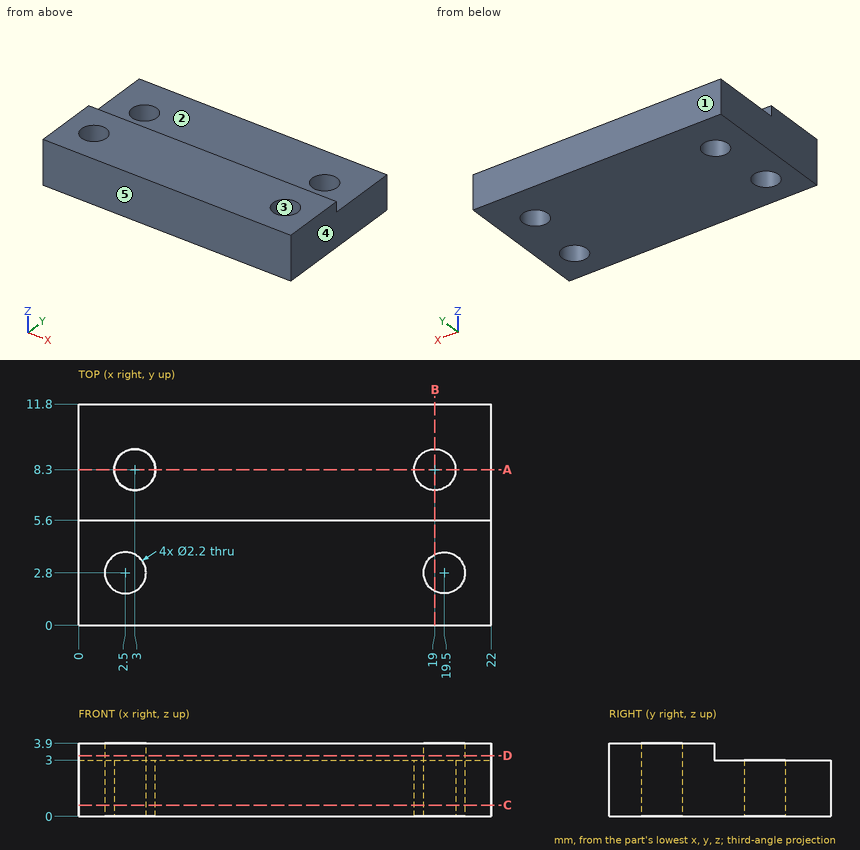
Design review of the part shown in the three views and the two pictorial views. Dimensions are in mm from the part's minimum x, y and z. A direction names the side the tool comes from. Round coordinates to 2 decimals unless told otherwise and drop trailing zeros. Write each loop counter-clockwise with the first axis right and the second up, starting at its lowest first coordinate (ties: lowest second). Pieces come first, ordered by that corner, then holes. Notation, with made-up numbers: M 40.25,86 L 50.25,86 A24 cw 50.25,119 Z; hole C 54,17 d6. An arc over 180 degrees is marked long. Use a Markdown table: item, result. Add a question column.
Q1. The part is to be moulded in two halves that separate along X. For the marked faces 3, 4 and 5, say which applies: pulls with the +X half, pulls with the -X half, needs draft (parallel to the pull), parting line crosses it, or undercut.
Q2. We need section B-B, the plane x = 19. State the section outline as (y, z) points, plus the area to 3 significant figures.
Q3. We need section A-A, the plane y = 8.3. State the section outline as (x, z) points, plus the area to 3 significant figures.
Q4. To check wall thickness, follow line 1 (Y direction, x = 19, z = 0.7); line 2 (Z direction, x = 14.5, y = 9.25); line 3 (Y direction, x = 8, z = 3.5). State the ranges of each line that lie inside material, in increasing order.
Q5. We need section C-C, the plane z = 0.6. State the section outline as (x, y) points, plus the area to 3 significant figures.
Q6. We need section D-D, the plane z = 3.25. State the section outline as (x, y) points, plus the area to 3 significant figures.
Q7. Insertion check: pin 1 (2 mm diameter, centred on x = 7, y = 9, fed in from +Z). The pin has a flat end and moves straight along its axis. Give the tip position at first contact, or say it passes through.
Q8. Machinability: for the marked faces 1 and 2, which of the approach directions +Z, -Z, +X, -X, +Y, -Y give a long, thin tool a straight path to every point of the face, cutting with its end or side? Answer none if there is none.
Findings below:
| question | item | result |
|---|---|---|
| 1 | face 3 | undercut |
| 1 | face 4 | pulls with the +X half |
| 1 | face 5 | needs draft |
| 2 | outline | M 0,0 L 1.82,0 L 1.82,3.9 L 0,3.9 Z; M 3.78,0 L 7.2,0 L 7.2,3 L 5.6,3 L 5.6,3.9 L 3.78,3.9 Z; M 9.4,0 L 11.8,0 L 11.8,3 L 9.4,3 Z |
| 2 | area | 26.2 mm² |
| 3 | outline | M 0,0 L 1.9,0 L 1.9,3 L 0,3 Z; M 4.1,0 L 17.9,0 L 17.9,3 L 4.1,3 Z; M 20.1,0 L 22,0 L 22,3 L 20.1,3 Z |
| 3 | area | 52.8 mm² |
| 4 | line 1 | y = 0 to 1.82, 3.78 to 7.2, 9.4 to 11.8 |
| 4 | line 2 | z = 0 to 3 |
| 4 | line 3 | y = 0 to 5.6 |
| 5 | outline | M 0,0 L 22,0 L 22,11.8 L 0,11.8 Z; hole C 2.5,2.8 d2.2; hole C 3,8.3 d2.2; hole C 19,8.3 d2.2; hole C 19.5,2.8 d2.2 |
| 5 | area | 244 mm² |
| 6 | outline | M 0,0 L 22,0 L 22,5.6 L 0,5.6 Z; hole C 2.5,2.8 d2.2; hole C 19.5,2.8 d2.2 |
| 6 | area | 116 mm² |
| 7 | pin 1 | stops at z = 3 |
| 8 | face 1 | +Z, -Z, +X, -X, +Y |
| 8 | face 2 | +Z, +X, -X, +Y |
